Geometry check sheet. Reference: drawing and pictorial views, mm from the part's lowest x, y, z. Give positions to 0.01 mm unless a question says otherwise; leave off trailing zeros. Order: outer loops, then holes, each group sorted by start corner. A loop starts at its lowest first (then second) coordinate and runs counter-clockwise, first axis right, second up.
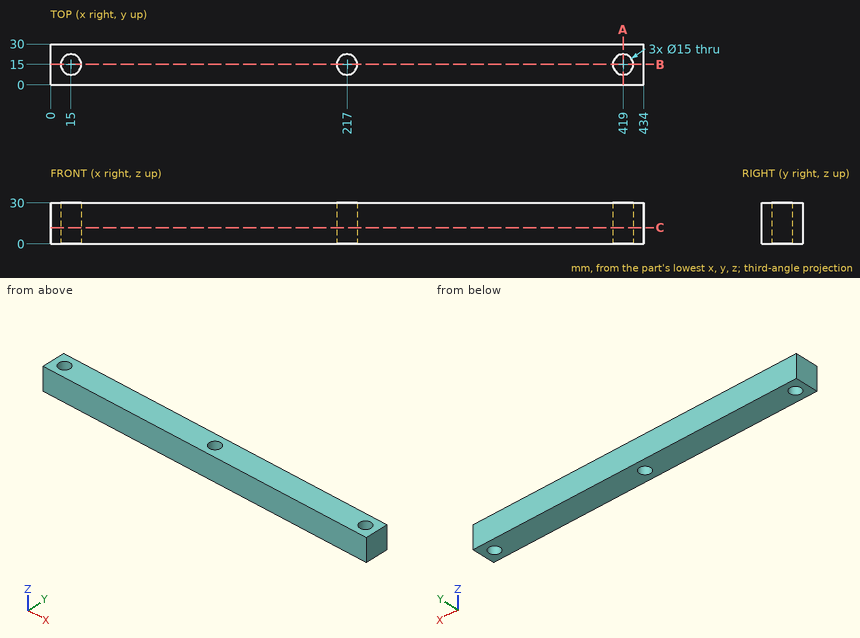
(1) Cross-section at B-B on y = 15. Enter the section's corners in (x, z).
Response values:
outline: (0, 0) - (7.5, 0) - (7.5, 30) - (0, 30) - close; (22.5, 0) - (209.5, 0) - (209.5, 30) - (22.5, 30) - close; (224.5, 0) - (411.5, 0) - (411.5, 30) - (224.5, 30) - close; (426.5, 0) - (434, 0) - (434, 30) - (426.5, 30) - close
(2) Cross-section at C-C on z = 12. Enter the section's corners in (x, y), then the cut area to 3 significant figures.
Response values:
outline: (0, 0) - (434, 0) - (434, 30) - (0, 30) - close; hole circle Ø15 at (15, 15); hole circle Ø15 at (217, 15); hole circle Ø15 at (419, 15)
area: 12,500 mm2
(3) Gauge pin test, flat end, axial feed: pin 1 Ø3 at (y, z) = (3.5, 15.5) entering from -X. Record the tip position at first contact, or that the pin passes through.
Response values:
pin 1: stops at x = 0
(4) Material ranges on L1, parallel to X at y = 14.5, z = 28.75; L2, parallel to X at y = 17.5, z = 16.25; L3, parallel to Y at x = 419, z = 18.25, recorded low to high.
Response values:
L1: x = 0 to 7.52, 22.48 to 209.52, 224.48 to 411.52, 426.48 to 434
L2: x = 0 to 7.93, 22.07 to 209.93, 224.07 to 411.93, 426.07 to 434
L3: y = 0 to 7.5, 22.5 to 30
(5) Cross-section at A-A on x = 419. Enter the section's corners in (y, z), then the cut area to 3 significant figures.
Response values:
outline: (0, 0) - (7.5, 0) - (7.5, 30) - (0, 30) - close; (22.5, 0) - (30, 0) - (30, 30) - (22.5, 30) - close
area: 450 mm2
